Input: part model. Units: mm. Frame: model coordinates. A direction names the side the tool comes from. Round coordinates to 2 decimals unless told otherwise and drop trailing zeros. Write each loop counter-clockwise with the first axis right and the second up, starting at its lowest first coordinate (ties: lowest second). Pieces come first, ordered by that corner, then holes. Notation, with made-up numbers: (6.25, 79.25) -> (28.25, 79.25) arc R29 ccw to (28.25, 100.25) -> close; hole circle Ø11 at (18, -27.5). An arc over 180 degrees is marked (long way). Use CSV: the item, a comma, the result in double quotes.
```python
from build123d import *

# Parameters (mm, degrees)
SKETCH2_R           = 0.9652
EXTRUDE1_DEPTH      = 5.0640001
EXTRUDE1_DEPTH_BACK = 5.0640001


with BuildPart() as part:
    # Sketch1 → Revolve Base (revolve)
    with BuildSketch(Plane(origin=(0, 0, 0), x_dir=(0, 0, -1), z_dir=(1, 0, 0))):
        with BuildLine():
            Line((0, 0), (0, 3.81))
            ThreePointArc((0, 3.81), (0.074394878, 3.989605122), (0.254, 4.064))
            Line((0.254, 4.064), (1.016, 4.064))
            ThreePointArc((1.016, 4.064), (1.105802561, 4.026802561), (1.143, 3.937))
            Line((1.143, 3.937), (1.143, 2.38125))
            Line((1.143, 2.38125), (12.8016, 2.38125))
            Line((12.8016, 2.38125), (13.1826, 2.00025))
            Line((13.1826, 2.00025), (13.1826, 0))
            Line((13.1826, 0), (0, 0))
        make_face()
    revolve(axis=Axis((0, 0, 0), (0, 0, -1)))

    # Sketch2 → Extrude1 (cut, two sides)
    with BuildSketch(Plane(origin=(0, 0, 0), x_dir=(0, 0, -1), z_dir=(1, 0, 0))) as extrude1_sk:
        with Locations((11.049, 0)):
            Circle(SKETCH2_R)
    extrude(amount=EXTRUDE1_DEPTH, mode=Mode.SUBTRACT)
    extrude(extrude1_sk.sketch, amount=-EXTRUDE1_DEPTH_BACK, mode=Mode.SUBTRACT)


solid = part.part
```
Item 1: Line query: line 1 (Z direction, x = -1.6, y = 0); line 2 (Z direction, x = 0.75, y = 3); line 3 (Z direction, x = -2, y = -0.5). Output: solid intervals per line, ascending.
Worked answers:
line 1,"z = -13.18 to -12.01, -10.08 to 0"
line 2,"z = -1.14 to 0"
line 3,"z = -13.12 to -11.87, -10.22 to 0"
Item 2: Section query A-A on y = 0. Return the cut outline in (x, z), plus the area to 3 significant figures.
Worked answers:
outline,"(-4.06, -1.02) arc R0.13 ccw to (-3.94, -1.14) -> (-2.38, -1.14) -> (-2.38, -10.08) -> (2.38, -10.08) -> (2.38, -1.14) -> (3.94, -1.14) arc R0.13 ccw to (4.06, -1.02) -> (4.06, -0.25) arc R0.25 ccw to (3.81, 0) -> (-3.81, 0) arc R0.25 ccw to (-4.06, -0.25) -> close; (-2.38, -12.8) -> (-2, -13.18) -> (2, -13.18) -> (2.38, -12.8) -> (2.38, -12.01) -> (-2.38, -12.01) -> close"
area,"57.3 mm²"
Item 3: First-contact query: pin 1 Ø1 at (x, z) = (-1.5, -4.5) entering from +Y; pin 2 Ø1.5 at (x, z) = (1.5, -6.5) entering from -Y; pin 3 Ø1.5 at (x, y) = (2, -2.5) entering from -Z. Flat tips, straight axial feed; report the tip coordinate or a pass-through.
Worked answers:
pin 1,"stops at y = 2.16"
pin 2,"stops at y = -2.26"
pin 3,"stops at z = -1.14"
Item 4: Set-up query: faces 1 (the face through (-2, 2, -1.143)), 2 (the face through (-3.967, -0.881, -0.64)). Return all of +Z, -Z, +X, -X, +Y, -Y with unobstructed straight access to the full face (end or side cutting, diameter ignored); none if empty.
Worked answers:
face 1,"-Z"
face 2,"+Z, -Z"
Item 5: Section query B-B on z = -11.5. Return the cut outline in (x, y), plus the area to 3 significant figures.
Worked answers:
outline,"(-2.22, -0.85) arc R2.38 ccw to (2.22, -0.85) -> close; (-2.22, 0.85) -> (2.22, 0.85) arc R2.38 ccw to start"
area,"9.86 mm²"
Item 6: Section query C-C on z = -7.5. Return the cut outline in (x, y).
Worked answers:
outline,"circle Ø4.76 at (0, 0)"
